CAD build for the part. Positions are in the model's coordinates, mm. A direction names the side the tool comes from. Round coordinates to 2 decimals unless told otherwise and drop trailing zeros. Loops run counter-clockwise (first coordinate to the right, second up) from the corner with the lowest first, then second, coordinate; pieces in that order, holes last.
from build123d import *

# Parameters (mm, degrees)
SKETCH2_R               = 3.75
BOSS_EXTRUDE1_DEPTH     = 6.5
SKETCH3_R               = 1.25
CUT_EXTRUDE1_DEPTH      = 1
CUT_EXTRUDE1_DEPTH_BACK = 7.5
SKETCH4_R               = 2.35
CUT_EXTRUDE2_DEPTH      = 1
CUT_EXTRUDE2_DEPTH_BACK = 1.5
SKETCH7_R               = 2.35
CUT_EXTRUDE5_DEPTH      = 3.4
SKETCH8_R               = 3.75
BOSS_EXTRUDE4_DEPTH     = 2.7


with BuildPart() as part:
    # Sketch2 → Boss-Extrude1 (new body)
    with BuildSketch(Plane(origin=(0, 0, 0), x_dir=(1, 0, 0), z_dir=(0, 1, 0))):
        Circle(SKETCH2_R)
    extrude(amount=BOSS_EXTRUDE1_DEPTH)

    # Sketch3 → Cut-Extrude1 (cut, two sides)
    with BuildSketch(Plane(origin=(0, 6.5, 0), x_dir=(1, 0, 0), z_dir=(0, 1, 0))) as cut_extrude1_sk:
        Circle(SKETCH3_R)
    extrude(amount=CUT_EXTRUDE1_DEPTH, mode=Mode.SUBTRACT)
    extrude(cut_extrude1_sk.sketch, amount=-CUT_EXTRUDE1_DEPTH_BACK, mode=Mode.SUBTRACT)

    # Sketch4 → Cut-Extrude2 (cut, two sides)
    with BuildSketch(Plane(origin=(0, 6.5, 0), x_dir=(1, 0, 0), z_dir=(0, 1, 0))) as cut_extrude2_sk:
        Circle(SKETCH4_R)
    extrude(amount=CUT_EXTRUDE2_DEPTH, mode=Mode.SUBTRACT)
    extrude(cut_extrude2_sk.sketch, amount=-CUT_EXTRUDE2_DEPTH_BACK, mode=Mode.SUBTRACT)

    # Sketch7 → Cut-Extrude5 (cut)
    with BuildSketch(Plane.XZ):
        Circle(SKETCH7_R)
    extrude(amount=-CUT_EXTRUDE5_DEPTH, mode=Mode.SUBTRACT)

    # Sketch8 → Boss-Extrude4 (add)
    with BuildSketch(Plane(origin=(0, 6, 0), x_dir=(1, 0, 0), z_dir=(0, 1, 0))):
        with BuildLine():
            Line((-9, -3.75), (-4.159026328, -3.75))
            ThreePointArc((-4.159026328, -3.75), (0, -5.6), (4.159026328, -3.75))
            Line((4.159026328, -3.75), (9, -3.75))
            Line((9, -3.75), (17.404544417, -2.445725053))
            ThreePointArc((17.404544417, -2.445725053), (19.5, 0), (17.404544417, 2.445725053))
            Line((17.404544417, 2.445725053), (9, 3.75))
            Line((9, 3.75), (4.159026328, 3.75))
            ThreePointArc((4.159026328, 3.75), (0, 5.6), (-4.159026328, 3.75))
            Line((-4.159026328, 3.75), (-9, 3.75))
            Line((-9, 3.75), (-17.404544417, 2.445725053))
            ThreePointArc((-17.404544417, 2.445725053), (-19.5, 0), (-17.404544417, -2.445725053))
            Line((-17.404544417, -2.445725053), (-9, -3.75))
        make_face()
        with BuildLine():
            ThreePointArc((-13.05, 0.75), (-12.3, 0), (-13.05, -0.75))
            Line((-13.05, -0.75), (-17.05, -0.75))
            ThreePointArc((-17.05, -0.75), (-17.8, 0), (-17.05, 0.75))
            Line((-17.05, 0.75), (-13.05, 0.75))
        make_face(mode=Mode.SUBTRACT)
        with BuildLine():
            ThreePointArc((-7, 0.75), (-6.25, 0), (-7, -0.75))
            Line((-7, -0.75), (-10.5, -0.75))
            ThreePointArc((-10.5, -0.75), (-11.25, 0), (-10.5, 0.75))
            Line((-10.5, 0.75), (-7, 0.75))
        make_face(mode=Mode.SUBTRACT)
        Circle(SKETCH8_R, mode=Mode.SUBTRACT)
        with BuildLine():
            ThreePointArc((7, -0.75), (6.25, 0), (7, 0.75))
            Line((7, 0.75), (10.5, 0.75))
            ThreePointArc((10.5, 0.75), (11.25, 0), (10.5, -0.75))
            Line((10.5, -0.75), (7, -0.75))
        make_face(mode=Mode.SUBTRACT)
        with BuildLine():
            ThreePointArc((17.05, 0.75), (17.8, 0), (17.05, -0.75))
            Line((17.05, -0.75), (13.05, -0.75))
            ThreePointArc((13.05, -0.75), (12.3, 0), (13.05, 0.75))
            Line((13.05, 0.75), (17.05, 0.75))
        make_face(mode=Mode.SUBTRACT)
    extrude(amount=-BOSS_EXTRUDE4_DEPTH)


solid = part.part
Item 1: Mould opens along Z. For faces 1 (the cylindrical face through (6.25, 4.67, 0.02)), 2 (the flat face through (-13.26, 4.67, 3.09)), 3 (the flat face through (13.26, 4.67, -3.09)) say: released by +Z, released by -Z, zero draft, split by the parting line, or undercut.
Verdict:
face 1: undercut
face 2: released by +Z
face 3: released by -Z
Item 2: Wall check: L1, parallel to Z at x = 0, y = 2.2; L2, parallel to Y at x = 5.5, z = 2; L3, parallel to X at y = 4.5, z = -0.25. Give the ranges that are in metal, low to high.
Verdict:
L1: z = -3.75 to -2.35, 2.35 to 3.75
L2: y = 3.3 to 6
L3: x = -19.49 to -17.76, -12.34 to -11.21, -6.29 to -1.22, 1.22 to 6.29, 11.21 to 12.34, 17.76 to 19.49
Item 3: Cut at A-A (x = 0). List the corners of the cut face in (y, z), plus the area to 3 significant figures.
Verdict:
outline: (0, -3.75) - (3.3, -3.75) - (3.3, -5.6) - (6, -5.6) - (6, -3.75) - (6.5, -3.75) - (6.5, -2.35) - (5, -2.35) - (5, -1.25) - (3.4, -1.25) - (3.4, -2.35) - (0, -2.35) - close; (0, 2.35) - (3.4, 2.35) - (3.4, 1.25) - (5, 1.25) - (5, 2.35) - (6.5, 2.35) - (6.5, 3.75) - (6, 3.75) - (6, 5.6) - (3.3, 5.6) - (3.3, 3.75) - (0, 3.75) - close
area: 31.7 mm2
Item 4: Flat gauge pins, fed straight in: P1, Ø0.8, axis at x = 15, y = 4.5, coming from the -Z side; P2, Ø1.4, axis at x = -14, y = 4.5, coming from the +Z side; P3, Ø0.8, axis at x = -14.5, y = 5, coming from the -Z side. Where does each tip first touch, or does it go through?
Verdict:
P1: stops at z = -2.88
P2: stops at z = 3.08
P3: stops at z = -2.96
Item 5: 3-axis set-ups, long thin cutter, end or side, ignore diameter. For faces 4 (the cylindrical face through (12.3, 4.7, 0)), 5 (the flat face through (7, 5, 3.75)), 6 (the cylindrical face through (-0.509, 5.76, 2.294)), 7 (the flat face through (-7, 5, 3.75)): which of +Z, -Z, +X, -X, +Y, -Y reach the whole face in a straight line?
Verdict:
face 4: +Y, -Y
face 5: +Z, +X, +Y, -Y
face 6: +Y
face 7: +Z, -X, +Y, -Y
Item 6: Cut at B-B (y = 4.25). State how many separate pieces and enclosed holes the cut face has, plus the area to 3 significant figures.
Verdict:
separate pieces: 1
enclosed holes: 5
area: 241 mm2
Item 7: Cut at C-C (y = 2.5). List the corners of the cut face in (x, z), plus the area to 3 significant figures.
Verdict:
outline: circle Ø7.5 at (0, 0); hole circle Ø4.7 at (0, 0)
area: 26.8 mm2
